Check sheet for the drawn part. Datum: minimum x, y, z corner. Units: mm. A direction names the side the tool comes from. Coordinates: 2 decimals unless noted, no trailing zeros. Write each loop counter-clockwise with the first axis right and the second up, starting at its lowest first coordinate (ties: lowest second). Pieces come first, ordered by that corner, then holes. Notation, with made-up numbers: (10, 67.5) -> (23, 67.5) arc R16 ccw to (23, 97.5) -> close; hole circle Ø3 at (15, -23). An arc over 180 degrees is marked (long way). Answer in a Markdown table with one row per item. Add a question column.
Q1. Tool access check on the marked faces 1 and 2. Record the directions out of +Z, -Z, +X, -X, +Y, -Y that give a thin tool (end or side, any length) a straight path to the whole face; none if there is none.
Q2. Section check B-B, the plane z = 1.75. Record the boundary of the cut face in (x, y), and give its area (3 significant figures).
Q3. Section check A-A, the plane z = 5.5. Record the boundary of the cut face in (x, y), and give its area (3 significant figures).
Q4. Thickness scan on line 1 (Z direction, x = 4, y = 7); line 2 (Z direction, x = 12.25, y = 12.25); line 3 (X direction, y = 7.25, z = 3.75). Record the ranges inside material, lowest first.
Q5. Gauge pin test, flat ends, axial feed: P1, Ø3, axis at x = 8.5, z = 1.5, coming from the -Y side; P2, Ø6, axis at x = 2.5, y = 6.5, coming from the -Z side; P3, Ø2, axis at x = 8.5, z = 2, coming from the +Y side. Record the tip position at first contact, or that the pin passes through.
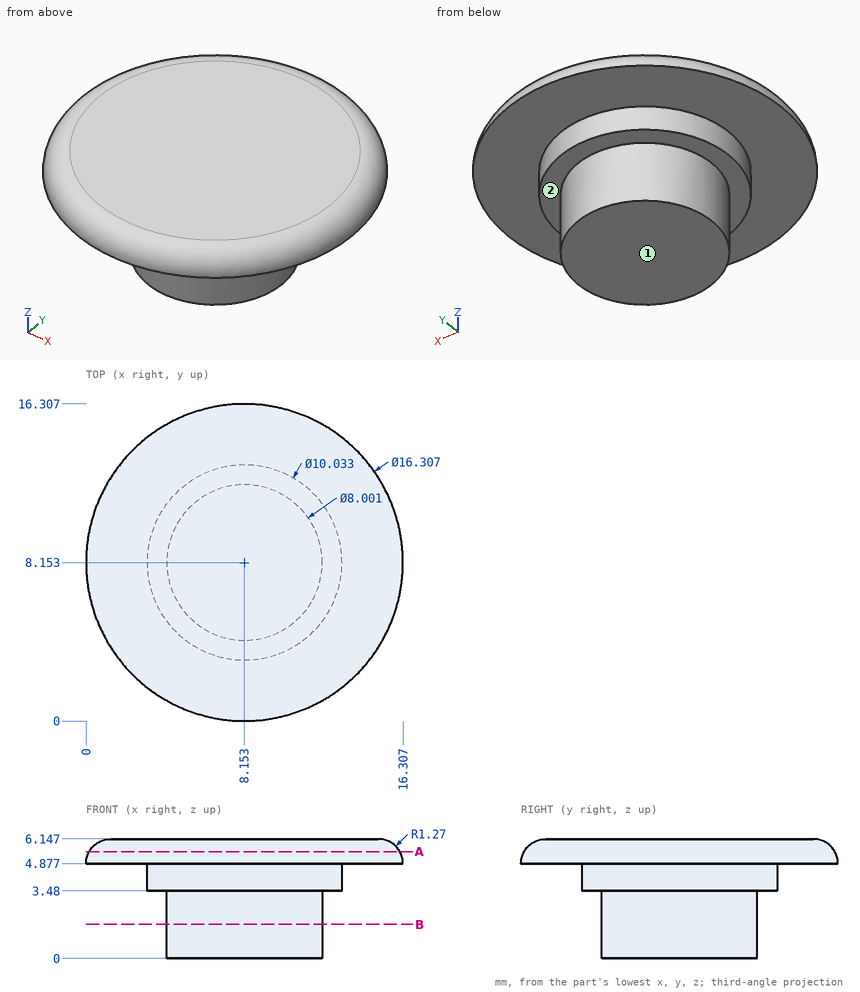
Calculated:
| question | item | result |
|---|---|---|
| 1 | face 1 | -Z, +X, -X, +Y, -Y |
| 1 | face 2 | -Z |
| 2 | outline | circle Ø8 at (8.15, 8.15) |
| 2 | area | 50.3 mm² |
| 3 | outline | circle Ø15.98 at (8.15, 8.15) |
| 3 | area | 201 mm² |
| 4 | line 1 | z = 3.48 to 6.15 |
| 4 | line 2 | z = 4.88 to 6.15 |
| 4 | line 3 | x = 3.22 to 13.09 |
| 5 | P1 | stops at y = 4.15 |
| 5 | P2 | stops at z = 0 |
| 5 | P3 | stops at y = 12.15 |
